from build123d import *

# Parameters (mm, degrees)
SKETCH1_W           = 40
SKETCH1_H           = 40
SKETCH1_W_2         = 24
SKETCH1_H_2         = 24
BOSS_EXTRUDE1_DEPTH = 40
SKETCH2_R           = 18
BOSS_EXTRUDE3_DEPTH = 30
SKETCH3_R           = 9
CUT_EXTRUDE1_DEPTH  = 62


with BuildPart() as part:
    # Sketch1 → Boss-Extrude1 (new body)
    with BuildSketch(Plane.XY):
        Rectangle(SKETCH1_W, SKETCH1_H)
        Rectangle(SKETCH1_W_2, SKETCH1_H_2, mode=Mode.SUBTRACT)
    extrude(amount=BOSS_EXTRUDE1_DEPTH)

    # Sketch2 → Boss-Extrude3 (add)
    with BuildSketch(Plane.ZY.offset(20)):
        with Locations(Location((20, 0, 0), (0, 0, 270))):
            Circle(SKETCH2_R)
    boss_extrude3 = extrude(amount=BOSS_EXTRUDE3_DEPTH)

    # Sketch3 → Cut-Extrude1 (cut)
    with BuildSketch(Plane.ZY.offset(50)):
        with Locations(Location((20, 0, 0), (0, 0, 270))):
            Circle(SKETCH3_R)
    cut_extrude1 = extrude(amount=-CUT_EXTRUDE1_DEPTH, mode=Mode.SUBTRACT)

    # Mirror1: Boss-Extrude3, Cut-Extrude1 across plane
    add(boss_extrude3.mirror(Plane(origin=(0, 0, 0), x_dir=(0, 0, 1), z_dir=(1, 0, 0))))
    add(cut_extrude1.mirror(Plane(origin=(0, 0, 0), x_dir=(0, 0, 1), z_dir=(1, 0, 0))), mode=Mode.SUBTRACT)


solid = part.part
Verification items for the finished model (mm, model axes). A direction names the side the tool comes from. Give positions to 0.01 mm unless a question says otherwise; leave off trailing zeros. Order: outer loops, then holes, each group sorted by start corner. A loop starts at its lowest first (then second) coordinate and runs counter-clockwise, first axis right, second up. Notation, with made-up numbers: M -23,13 L 30,13 A14 ccw 30,18 Z; hole C 58.5,-29 d11. An arc over 180 degrees is marked long. Use one line per item in the form item = value. Start each with the question number.
Q1. Section check C-C (y = 0). Enter the section's corners in (x, z).
Q2. Access from +Z, -Z, +X, -X, +Y, -Y to the whole of each face (thin tool, end or side, straight path). Record for faces 4 (the flat face through (0, 20, 20)), 5 (the flat face through (12, -0.2, 10.8)), 6 (the cylindrical face through (34.79, 3.902, 2.428)), 7 (the cylindrical face through (-34.79, 3.902, 2.428)).
Q3. Mould release check, pull along X, two halves, no side actions. Record for faces 1 (the flat face through (-12, -0.2, 10.8)), 2 (the flat face through (-20, -5, 2)), 3 (the cylindrical face through (-31.266, 1.172, 28.923)): +X half, -X half, draft (parallel to the pull), parting line (faces both ways), or undercut.
Q4. Section check A-A (x = -7). Enter the section's corners in (y, z).
Q5. Section check B-B (z = 20). Enter the section's corners in (x, y), then the cut area to 3 significant figures.
Q6. Scan lines: line 1 along X through (y, z) = (7, 13); line 2 along Z through (x, y) = (33.5, 0); line 3 along X through (y, z) = (-10, 35). Record each from-to range of solid material in increasing order. Write a range as [from, to].
Q7. Section check D-D (x = 18). Enter the section's corners in (y, z), then the cut area to 3 significant figures.
Q8. Go/stop test with flat-tipped pins: pin 1 Ø4 at (x, y) = (40, -1.5) entering from +Z; pin 2 Ø4 at (x, z) = (24, 21.5) entering from +Y; pin 3 Ø5 at (x, z) = (-40, 33) entering from -Y. Record where each tip stops, or that it passes through.
Evaluation:
q1.outline = M -50,2 L -20,2 L -20,0 L -12,0 L -12,11 L -50,11 Z; M -50,29 L -12,29 L -12,40 L -20,40 L -20,38 L -50,38 Z; M 12,0 L 20,0 L 20,2 L 50,2 L 50,11 L 12,11 Z; M 12,29 L 50,29 L 50,38 L 20,38 L 20,40 L 12,40 Z
q2.face_4 = +Z, -Z, +X, -X, +Y
q2.face_5 = +Z, -Z
q2.face_6 = +X
q2.face_7 = -X
q3.face_1 = undercut
q3.face_2 = -X half
q3.face_3 = draft
q4.outline = M -20,0 L -12,0 L -12,40 L -20,40 Z; M 12,0 L 20,0 L 20,40 L 12,40 Z
q5.outline = M -50,-18 L -20,-18 L -20,-20 L 20,-20 L 20,-18 L 50,-18 L 50,-9 L 12,-9 L 12,-12 L -12,-12 L -12,-9 L -50,-9 Z; M -50,9 L -12,9 L -12,12 L 12,12 L 12,9 L 50,9 L 50,18 L 20,18 L 20,20 L -20,20 L -20,18 L -50,18 Z
q5.area = 1,820 mm2
q6.line_1 = [-50, -12], [12, 50]
q6.line_2 = [2, 11], [29, 38]
q6.line_3 = [-20, -12], [12, 20]
q7.outline = M -20,0 L 20,0 L 20,40 L -20,40 Z; hole C 0,20 d18
q7.area = 1,350 mm2
q8.pin_1 = 38
q8.pin_2 = 18
q8.pin_3 = -14.62
